Autodesk Inventor part; units mm, degrees
ref_plane "YZ Plane" through (0, 0, 0) normal (1, 0, 0) x (0, 1, 0)
ref_plane "XZ Plane" through (0, 0, 0) normal (0, 1, 0) x (-1, 0, 0)
ref_plane "XY Plane" through (0, 0, 0) normal (0, 0, 1) x (1, 0, 0)
sketch "Sketch1" plane through (0, 0, 0) normal (0, 0, 1) x (1, 0, 0)
  line L0 (-122.1855, 0) -> (62.4119, 0)
  line L1 (0, -27.4264) -> (0, 36.5685)
  circle A0 centre (0, 0) radius 6.5
  line L2 (-4.5, 20.5122) -> (-4.5, 14.3091)
  line L3 (-20.5122, 4.5) -> (-14.3091, 4.5)
  line L4 (4.5, -14.3091) -> (4.5, -20.5122)
  line L5 (20.5122, -4.5) -> (14.3091, -4.5)
  arc A1 (-4.5, 20.5122) -> (-20.5122, 4.5) centre (0, 0) ccw
  arc A2 (4.5, -20.5122) -> (20.5122, -4.5) centre (0, 0) ccw
  arc A3 (-4.5, 16.3936) -> (-16.3936, 4.5) centre (0, 0) ccw
  arc A4 (4.5, -16.3936) -> (16.3936, -4.5) centre (0, 0) ccw
  arc A5 (-14.3091, 4.5) -> (4.5, -14.3091) centre (0, 0) ccw
  arc A6 (14.3091, -4.5) -> (-4.5, 14.3091) centre (0, 0) ccw
  line L6 (-18.9737, 9) -> (-100, 9)
  arc A7 (-100, 9) -> (-100, -9) centre (-100, 0) ccw
  line L7 (-100, -9) -> (-12, -9)
  dimension "d0" = 13
  dimension "d1" = 30
  dimension "d2" = 34
  dimension "d3" = 42
  dimension "d4" = 4.5
  dimension "d5" = 4.5
  dimension "d6" = 100
  dimension "d7" = 9
extrude "Extrusion1" add sketch "Sketch1" along normal mid plane 9 contours A7 L6 A1 L3 A5 L0 | L0 A5 L7 A7 | A5 L3 A3 L2 A6 L1 A0 L0 | L0 A0 L1 A5 | L1 A6 L0 A0 | A0 L0 A6 L5 A4 L4 A5 L1
extrude "Extrusion2" add sketch "Sketch1" along normal mid plane 22 contours A1 L2 A3 L3 | A4 L5 A2 L4
sketch "Sketch2" plane through (0, 0, 0) normal (0, 1, 0) x (-1, 0, 0)
  line L0 (2.4, 0) -> (-3.2, 0)
  line L1 (0, -2.4) -> (0, 3.2)
  circle A0 centre (0, 0) radius 2
  dimension "d12" = 4
extrude "Extrusion3" cut sketch "Sketch2" along normal through all both and the other way through all
properties part number "Handle" material "Steel, Mild"
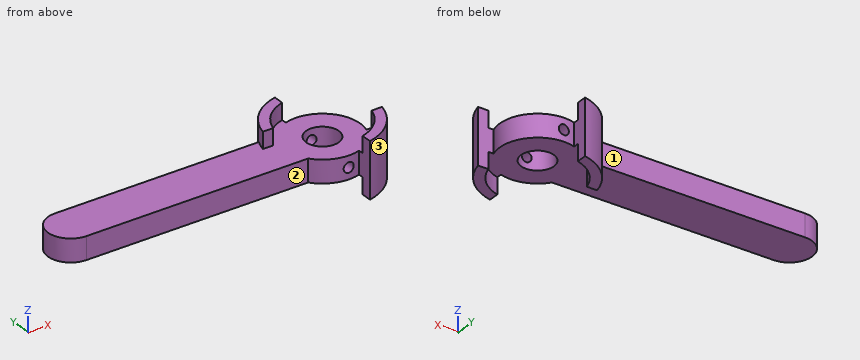
Check sheet for the modelled part. Datum: model origin and axes. Units: mm. Face numbers are marked on the shaded views. A direction names the side the tool comes from. Round coordinates to 2 decimals unless told otherwise and drop trailing zeros. Order: outer loops, then holes, each group sorted by start corner. A loop starts at its lowest first (then second) coordinate and runs counter-clockwise, first axis right, second up. Notation, with made-up numbers: M 76,6.5 L 126,6.5 A27 cw 126,25.5 Z; hole C -14.5,-4 d3. An arc over 180 degrees is marked long. Answer in a Markdown table with one row per item.
(1) Section check C-C on x = -81. Record the boundary of the cut face in (y, z).
Findings:
| item | result |
|---|---|
| outline | M -9,-4.5 L 9,-4.5 L 9,4.5 L -9,4.5 Z |
(2) Gauge pin test, flat ends, axial feed: pin 1 (7 mm diameter, centred on x = -40.5, z = 0.5, fed in from +Y); pin 2 (3 mm diameter, centred on y = -19, z = -4.5, fed in from -X); pin 3 (10 mm diameter, centred on x = -43.5, z = -5.5, fed in from -Y); pin 4 (3.5 mm diameter, centred on x = 0, z = 0, fed in from +Y). Record the tip position at first contact, or that the pin passes through.
Findings:
| item | result |
|---|---|
| pin 1 | stops at y = 9 |
| pin 2 | stops at x = 4.5 |
| pin 3 | stops at y = -9 |
| pin 4 | passes through |
(3) Section check B-B on z = -7. Record the boundary of the cut face in (x, y).
Findings:
| item | result |
|---|---|
| outline | M -20.51,4.5 L -16.39,4.5 A17 cw -4.5,16.39 L -4.5,20.51 A21 ccw Z; M 4.5,-20.51 A21 ccw 20.51,-4.5 L 16.39,-4.5 A17 cw 4.5,-16.39 Z |
(4) Section check D-D on z = 0. Record the boundary of the cut face in (x, y), plus the area to 3 significant figures.
Findings:
| item | result |
|---|---|
| outline | M -100,-9 L -12,-9 A15 ccw -2,-14.87 L -2,-6.18 A6.5 cw -2,6.18 L -2,14.87 A15 ccw -4.5,14.31 L -4.5,20.51 A21 ccw -18.97,9 L -100,9 A9 ccw Z; M 2,-14.87 A15 ccw 4.5,-14.31 L 4.5,-20.51 A21 ccw 20.51,-4.5 L 14.31,-4.5 A15 ccw 2,14.87 L 2,6.18 A6.5 cw 2,-6.18 Z |
| area | 2,380 mm^2 |
(5) Material ranges on line 1 along Z through (x, y) = (0, -12); line 2 along X through (y, z) = (0, 0.5); line 3 along Z through (x, y) = (-10, -11), recorded low to high. Write a range as from..to.
Findings:
| item | result |
|---|---|
| line 1 | z = -4.5..-2, 2..4.5 |
| line 2 | x = -109..-6.5, 6.5..15 |
| line 3 | z = -4.5..4.5 |
(6) Set-up check for the marked faces 1, 2 and 3: record each of +Z, -Z, +X, -X, +Y, -Y from which the full face is reachable in a straight line by a thin tool's end or side.
Findings:
| item | result |
|---|---|
| face 1 | +Z, -Z, -X, +Y |
| face 2 | +Z, -Z, -X, -Y |
| face 3 | +Z, -Z, +X, -Y |
(7) Section check A-A on x = 0. Record the boundary of the cut face in (y, z).
Findings:
| item | result |
|---|---|
| outline | M -15,-4.5 L -6.5,-4.5 L -6.5,-2 L -15,-2 Z; M -15,2 L -6.5,2 L -6.5,4.5 L -15,4.5 Z; M 6.5,-4.5 L 15,-4.5 L 15,-2 L 6.5,-2 Z; M 6.5,2 L 15,2 L 15,4.5 L 6.5,4.5 Z |
